Design review of the part built by this model. Coordinates are the model's own, in mm. Face numbers are marked on the shaded views. A direction names the side the tool comes from. Give positions to 0.01 mm unless a question says otherwise; leave off trailing zeros. Loops run counter-clockwise (first coordinate to the right, second up) from the corner with the lowest first, then second, coordinate; pieces in that order, holes last. Notation, with made-up numbers: M 25.5,-4.75 L 39.5,-4.75 A20 cw 39.5,25.25 Z; hole C -31.5,35 d4. An arc over 180 degrees is marked long. Use one line per item in the form item = value. Start each with the question number.
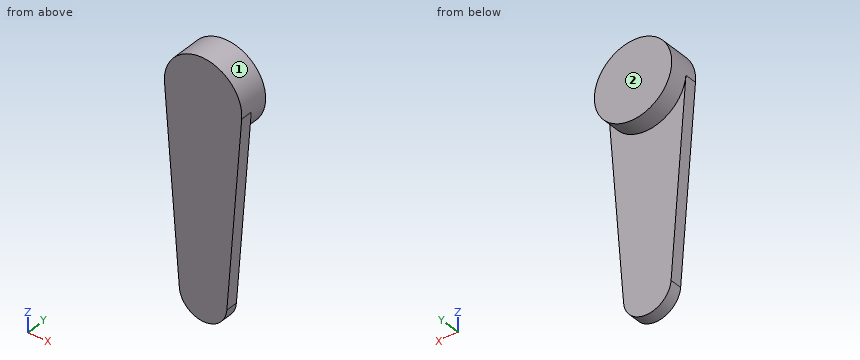
Autodesk Inventor part; units mm, degrees
ref_plane "YZ Plane" through (0, 0, 0) normal (1, 0, 0) x (0, 1, 0)
ref_plane "XZ Plane" through (0, 0, 0) normal (0, 1, 0) x (-1, 0, 0)
ref_plane "XY Plane" through (0, 0, 0) normal (0, 0, 1) x (1, 0, 0)
sketch "Sketch1" plane through (0, 0, 0) normal (0, 1, 0) x (-1, 0, 0)
  circle A0 centre (0, 0) radius 3.25
  circle A1 centre (0, -16.25) radius 2
  line L0 (3.2404, -0.25) -> (1.9941, -16.4038)
  line L1 (-1.9941, -16.4038) -> (-3.2404, -0.25)
  dimension "d0" = 6.5
  dimension "d1" = 4
  dimension "d2" = 21.5
extrude "Extrusion1" add sketch "Sketch1" along normal blind 1
extrude "Extrusion2" add sketch "Sketch1" along normal blind 2.5 contours A0
properties part number "Servo attachment"
Q1. Take a section at C-C on z = -10.75. Give the boundary of the cut face in (x, y), plus the area to 3 significant figures.
Q2. Clearance check with flat-ended pins moving along their axes: pin 1 Ø1.9 at (x, z) = (1, -9) entering from +Y; pin 2 Ø1.5 at (x, y) = (-1, 1.5) entering from +Z. State where each tip first meets the part, or that it passes through.
Q3. Take a section at B-B on y = 2. Give the boundary of the cut face in (x, z), plus the area to 3 significant figures.
Q4. Take a section at D-D on x = 1.25. Give the boundary of the cut face in (y, z), plus the area to 3 significant figures.
Q5. Take a section at A-A on x = 0. Give the boundary of the cut face in (y, z), plus the area to 4 significant figures.
Q6. Wall thickness on probe 1 along Z at (x, y) = (0.25, 1.45); probe 2 along Y at (x, z) = (-2.75, -2); probe 3 along Z at (x, y) = (2.25, 2.25): over which ranges is each line inside the solid? List them lowest first.
Q7. For the marked faces 1 and 2, list the 3-axis set-ups (+Z, -Z, +X, -X, +Y, -Y) from which the entire face can be reached by the end or side of a thin tool; tool diameter is ignored.
Response values:
q1.outline = M -2.43,0 L 2.43,0 L 2.43,1 L -2.43,1 Z
q1.area = 4.86 mm^2
q2.pin_1 = 1
q2.pin_2 = 3.24
q3.outline = C 0,0 d6.5
q3.area = 33.2 mm^2
q4.outline = M 0,-17.81 L 1,-17.81 L 1,-3 L 2.5,-3 L 2.5,3 L 0,3 Z
q4.area = 29.8 mm^2
q5.outline = M 0,-18.25 L 1,-18.25 L 1,-3.25 L 2.5,-3.25 L 2.5,3.25 L 0,3.25 Z
q5.area = 31.25 mm^2
q6.probe_1 = -3.24 to 3.24
q6.probe_2 = 0 to 1
q6.probe_3 = -2.35 to 2.35
q7.face_1 = +Y
q7.face_2 = +Z, -Z, +X, -X, +Y
